Can you work these out from the model? Positions are in its coordinate system, mm. A direction names the side the tool comes from. Give positions to 0.01 mm unless a question says otherwise; leave off trailing zeros. Loops run counter-clockwise (first coordinate to the right, second up) from the corner with the lowest first, then second, coordinate; pieces in that order, holes last. Notation, with made-up numbers: (12, 8.5) - (35, 8.5) arc R20 cw to (35, 14.5) - close; hole circle Ø1 at (55.5, 32). An arc over 180 degrees is marked (long way). Answer in a Markdown table with one row per item.
from build123d import *

# Parameters (mm, degrees)
SKETCH1_W                                    = 130.62
SKETCH1_H                                    = 3
SKETCH1_W_2                                  = 18.99
SKETCH1_W_3                                  = 25.43
SKETCH1_W_4                                  = 84.2
SKETCH1_H_2                                  = 2.79860344
BOSS_EXTRUDE1_DEPTH                          = 2
SKETCH2_W                                    = 130.62
SKETCH2_H                                    = 178.45860344
BOSS_EXTRUDE2_DEPTH                          = 3
CSK_FOR_M3_COUNTERSUNK_FLAT_HEAD_SCR_2_COUNT = 2
CSK_FOR_M3_COUNTERSUNK_FLAT_HEAD_SCR_2_PITCH = 53.025276991
CSK_FOR_M3_COUNTERSUNK_FLAT_HEAD_SCR_3_COUNT = 2
CSK_FOR_M3_COUNTERSUNK_FLAT_HEAD_SCR_3_PITCH = 66.620192134
CSK_FOR_M3_COUNTERSUNK_FLAT_HEAD_SCR_4_COUNT = 2
CSK_FOR_M3_COUNTERSUNK_FLAT_HEAD_SCR_4_PITCH = 48.217527933
SKETCH9_W                                    = 2.047760895
SKETCH9_H                                    = 53.7
SKETCH9_W_2                                  = 2
BOSS_EXTRUDE3_DEPTH                          = 24
SKETCH10_W                                   = 130.62
SKETCH10_H                                   = 3
BOSS_EXTRUDE4_DEPTH                          = 22
CUT_EXTRUDE1_DEPTH                           = 22
BOSS_EXTRUDE5_DEPTH                          = 22
SKETCH13_R                                   = 2
BOSS_EXTRUDE6_DEPTH                          = 24.5
SKETCH15_W                                   = 126.572239105
SKETCH15_H                                   = 3
SKETCH15_W_2                                 = 2
SKETCH15_H_2                                 = 172.45860344
SKETCH15_W_3                                 = 2.047760895
BOSS_EXTRUDE7_DEPTH                          = 2.5


with BuildPart() as part:
    # Sketch1 → Boss-Extrude1 (new body)
    with BuildSketch(Plane(origin=(0, 0, 0), x_dir=(1, 0, 0), z_dir=(0, 1, 0))):
        with Locations((69.266788991, -134.782980897)):
            Rectangle(SKETCH1_W, SKETCH1_H)
        with Locations((69.266788991, -78.082980897)):
            Rectangle(SKETCH1_W, SKETCH1_H)
        Polygon((134.576788991, -20.082980897), (109.146788991, -20.082980897), (109.146788991, -67.500327372), (109.146788991, -76.582980897), (134.576788991, -76.582980897), align=None)
        Polygon((22.946788991, -33.891997438), (22.946788991, -20.082980897), (3.956788991, -20.082980897), (3.956788991, -76.582980897), (22.946788991, -76.582980897), align=None)
        Polygon((22.946788991, -17.082980897), (22.946788991, 39.175622543), (6.956788991, 39.175622543), (3.956788991, 39.175622543), (3.956788991, -17.082980897), align=None)
        Polygon((131.576788991, 39.175622543), (109.146788991, 39.175622543), (109.146788991, -17.082980897), (134.576788991, -17.082980897), (134.576788991, 39.175622543), align=None)
        with Locations((13.451788991, -18.582980897)):
            Rectangle(SKETCH1_W_2, SKETCH1_H)
        with Locations((121.861788991, -18.582980897)):
            Rectangle(SKETCH1_W_3, SKETCH1_H)
        with Locations((66.046788991, -18.683679177)):
            Rectangle(SKETCH1_W_4, SKETCH1_H_2)
        Polygon((23.946788991, 39.175622543), (108.146788991, 39.175622543), (109.146788991, 39.175622543), (131.576788991, 39.175622543), (134.576788991, 39.175622543), (134.576788991, 42.175622543), (3.956788991, 42.175622543), (3.956788991, 39.175622543), (6.956788991, 39.175622543), (22.946788991, 39.175622543), align=None)
    extrude(amount=BOSS_EXTRUDE1_DEPTH)

    # Sketch2 → Boss-Extrude2 (add)
    with BuildSketch(Plane.XZ):
        with Locations((69.266788991, 47.053679177)):
            Rectangle(SKETCH2_W, SKETCH2_H)
    extrude(amount=BOSS_EXTRUDE2_DEPTH)

    # Sketch8 → CSK for M3 Countersunk Flat Head Screw1 (revolve, cut)
    with BuildSketch(Plane(origin=(88.234088991, 0, 130.282980897), x_dir=(0, 0, 1), z_dir=(1, 0, 0))):
        Polygon((0, 0), (0, 3), (1.7, 3), (1.7, 1.45), (3.15, 0), align=None)
    csk_for_m3_countersunk_flat_head_screw1 = revolve(axis=Axis((88.234088991, 6.35, 130.282980897), (0, -1, 0)), mode=Mode.SUBTRACT)

    # CSK for M3 Countersunk Flat Head Scr 2: CSK for M3 Countersunk Flat Head Screw1 ×2
    with Locations(*[Vector(-0.958033656445997, 0, -0.2866557397239995) * (i * CSK_FOR_M3_COUNTERSUNK_FLAT_HEAD_SCR_2_PITCH) for i in range(1, CSK_FOR_M3_COUNTERSUNK_FLAT_HEAD_SCR_2_COUNT)]):
        add(csk_for_m3_countersunk_flat_head_screw1, mode=Mode.SUBTRACT)

    # CSK for M3 Countersunk Flat Head Scr 3: CSK for M3 Countersunk Flat Head Screw1 ×2
    with Locations(*[Vector(-0.762531574476027, 0, -0.6469510011794644) * (i * CSK_FOR_M3_COUNTERSUNK_FLAT_HEAD_SCR_3_PITCH) for i in range(1, CSK_FOR_M3_COUNTERSUNK_FLAT_HEAD_SCR_3_COUNT)]):
        add(csk_for_m3_countersunk_flat_head_screw1, mode=Mode.SUBTRACT)

    # CSK for M3 Countersunk Flat Head Scr 4: CSK for M3 Countersunk Flat Head Screw1 ×2
    with Locations(*[Vector(0.02696114993281913, 0, -0.9996364821245272) * (i * CSK_FOR_M3_COUNTERSUNK_FLAT_HEAD_SCR_4_PITCH) for i in range(1, CSK_FOR_M3_COUNTERSUNK_FLAT_HEAD_SCR_4_COUNT)]):
        add(csk_for_m3_countersunk_flat_head_screw1, mode=Mode.SUBTRACT)

    # Sketch9 → Boss-Extrude3 (add)
    with BuildSketch(Plane(origin=(0, 0, 0), x_dir=(1, 0, 0), z_dir=(0, 1, 0))):
        with Locations((133.552908543, -106.432980897)):
            Rectangle(SKETCH9_W, SKETCH9_H)
        with Locations((4.956788991, -106.432980897)):
            Rectangle(SKETCH9_W_2, SKETCH9_H)
    extrude(amount=BOSS_EXTRUDE3_DEPTH)

    # Sketch10 → Boss-Extrude4 (add)
    with BuildSketch(Plane(origin=(0, 2, 0), x_dir=(1, 0, 0), z_dir=(0, 1, 0))):
        with Locations((69.266788991, -134.782980897)):
            Rectangle(SKETCH10_W, SKETCH10_H)
    extrude(amount=BOSS_EXTRUDE4_DEPTH)

    # Sketch11 → Cut-Extrude1 (cut)
    with BuildSketch(Plane(origin=(134.576788991, 0, 0), x_dir=(0, 0, -1), z_dir=(1, 0, 0))):
        with BuildLine():
            Line((-126.332980897, 2), (-107.932980897, 2))
            Line((-107.932980897, 2), (-107.932980897, 12))
            Line((-107.932980897, 12), (-123.378368558, 12))
            ThreePointArc((-123.378368558, 12), (-125.578874654, 7.213677543), (-126.332980897, 2))
        make_face()
        with BuildLine():
            Line((-107.932980897, 2), (-89.532980897, 2))
            ThreePointArc((-89.532980897, 2), (-90.28708714, 7.213677543), (-92.487593236, 12))
            Line((-92.487593236, 12), (-107.932980897, 12))
            Line((-107.932980897, 12), (-107.932980897, 2))
        make_face()
    extrude(amount=-CUT_EXTRUDE1_DEPTH, mode=Mode.SUBTRACT)

    # Sketch12 → Boss-Extrude5 (add)
    with BuildSketch(Plane(origin=(0, 2, 0), x_dir=(1, 0, 0), z_dir=(0, 1, 0))):
        Polygon((134.576788991, 42.175622543), (3.956788991, 42.175622543), (3.956788991, -79.582980897), (5.956788991, -79.582980897), (5.956788991, 39.175622543), (132.529028096, 39.175622543), (132.529028096, -79.582980897), (134.576788991, -79.582980897), align=None)
    extrude(amount=BOSS_EXTRUDE5_DEPTH)

    # Sketch13 → Boss-Extrude6 (add)
    with BuildSketch(Plane(origin=(0, 0, 0), x_dir=(1, 0, 0), z_dir=(0, 1, 0))):
        with BuildLine():
            Line((125.229028096, -117.857980897), (125.229028096, -119.857980897))
            Line((125.229028096, -119.857980897), (125.229028096, -121.857980897))
            ThreePointArc((125.229028096, -121.857980897), (126.643241659, -121.272194459), (127.229028096, -119.857980897))
            ThreePointArc((127.229028096, -119.857980897), (126.643241659, -118.443767335), (125.229028096, -117.857980897))
        make_face()
        with BuildLine():
            ThreePointArc((125.229028096, -117.857980897), (123.814814534, -118.443767335), (123.229028096, -119.857980897))
            Line((123.229028096, -119.857980897), (125.229028096, -119.857980897))
            Line((125.229028096, -119.857980897), (125.229028096, -117.857980897))
        make_face()
        with BuildLine():
            Line((125.229028096, -119.857980897), (123.229028096, -119.857980897))
            ThreePointArc((123.229028096, -119.857980897), (123.814814534, -121.272194459), (125.229028096, -121.857980897))
            Line((125.229028096, -121.857980897), (125.229028096, -119.857980897))
        make_face()
        with BuildLine():
            ThreePointArc((125.229028096, -117.857980897), (123.814814534, -118.443767335), (123.229028096, -119.857980897))
            Line((123.229028096, -119.857980897), (125.229028096, -119.857980897))
            Line((125.229028096, -119.857980897), (125.229028096, -117.857980897))
        make_face()
        with BuildLine():
            ThreePointArc((13.209288991, -121.857980897), (14.623502553, -121.272194459), (15.209288991, -119.857980897))
            Line((15.209288991, -119.857980897), (13.209288991, -119.857980897))
            Line((13.209288991, -119.857980897), (13.209288991, -121.857980897))
        make_face()
        with BuildLine():
            Line((13.209288991, -119.857980897), (15.209288991, -119.857980897))
            ThreePointArc((15.209288991, -119.857980897), (14.623502553, -118.443767335), (13.209288991, -117.857980897))
            Line((13.209288991, -117.857980897), (13.209288991, -119.857980897))
        make_face()
        with BuildLine():
            Line((13.209288991, -119.857980897), (15.209288991, -119.857980897))
            ThreePointArc((15.209288991, -119.857980897), (14.623502553, -118.443767335), (13.209288991, -117.857980897))
            Line((13.209288991, -117.857980897), (13.209288991, -119.857980897))
        make_face()
        with BuildLine():
            Line((13.209288991, -119.857980897), (13.209288991, -117.857980897))
            ThreePointArc((13.209288991, -117.857980897), (11.209288991, -119.857980897), (13.209288991, -121.857980897))
            Line((13.209288991, -121.857980897), (13.209288991, -119.857980897))
        make_face()
        with BuildLine():
            ThreePointArc((15.209288991, -93.007980897), (14.623502553, -91.593767335), (13.209288991, -91.007980897))
            Line((13.209288991, -91.007980897), (13.209288991, -93.007980897))
            Line((13.209288991, -93.007980897), (15.209288991, -93.007980897))
        make_face()
        with BuildLine():
            ThreePointArc((13.209288991, -95.007980897), (14.623502553, -94.422194459), (15.209288991, -93.007980897))
            Line((15.209288991, -93.007980897), (13.209288991, -93.007980897))
            Line((13.209288991, -93.007980897), (13.209288991, -95.007980897))
        make_face()
        with BuildLine():
            ThreePointArc((15.209288991, -93.007980897), (14.623502553, -91.593767335), (13.209288991, -91.007980897))
            Line((13.209288991, -91.007980897), (13.209288991, -93.007980897))
            Line((13.209288991, -93.007980897), (15.209288991, -93.007980897))
        make_face()
        with BuildLine():
            ThreePointArc((13.209288991, -95.007980897), (14.623502553, -94.422194459), (15.209288991, -93.007980897))
            Line((15.209288991, -93.007980897), (13.209288991, -93.007980897))
            Line((13.209288991, -93.007980897), (13.209288991, -95.007980897))
        make_face()
        with BuildLine():
            Line((13.209288991, -93.007980897), (13.209288991, -91.007980897))
            ThreePointArc((13.209288991, -91.007980897), (11.209288991, -93.007980897), (13.209288991, -95.007980897))
            Line((13.209288991, -95.007980897), (13.209288991, -93.007980897))
        make_face()
        with Locations(Location((125.229028096, -93.007980897, 0), (0, 0, 90))):
            Circle(SKETCH13_R)
    extrude(amount=BOSS_EXTRUDE6_DEPTH)

    # Sketch15 → Boss-Extrude7 (add)
    with BuildSketch(Plane(origin=(0, 24, 0), x_dir=(1, 0, 0), z_dir=(0, 1, 0))):
        with Locations((69.242908544, 40.675622543)):
            Rectangle(SKETCH15_W, SKETCH15_H)
        with Locations((4.956788991, -47.053679177)):
            Rectangle(SKETCH15_W_2, SKETCH15_H_2)
        with Locations((4.956788991, 40.675622543)):
            Rectangle(SKETCH15_W_2, SKETCH15_H)
        with Locations((133.552908543, 40.675622543)):
            Rectangle(SKETCH15_W_3, SKETCH15_H)
        Polygon((134.576788991, -136.282980897), (134.576788991, 39.175622543), (132.529028096, 39.175622543), (132.529028096, -133.282980897), (132.529028096, -136.282980897), align=None)
        with Locations((4.956788991, -134.782980897)):
            Rectangle(SKETCH15_W_2, SKETCH15_H)
        with Locations((69.242908544, -134.782980897)):
            Rectangle(SKETCH15_W, SKETCH15_H)
    extrude(amount=BOSS_EXTRUDE7_DEPTH)


solid = part.part
Q1. Imagine slicing it at B-B, the plane y = 16.5. Write out the boundary of the cut face in (x, z), and give its area (3 significant figures).
Checked values:
| item | result |
|---|---|
| outline | (3.96, -42.18) - (134.58, -42.18) - (134.58, 136.28) - (3.96, 136.28) - close; circle Ø4 at (13.21, 93.01); circle Ø4 at (13.21, 119.86); circle Ø4 at (125.23, 93.01); circle Ø4 at (125.23, 119.86); hole (5.96, -39.18) - (132.53, -39.18) - (132.53, 133.28) - (5.96, 133.28) - close |
| area | 1,530 mm² |
Q2. If we mould it in two halves opening along X, with no side actions, what happens to faces 3 (the face through (68, 13, -39.176)), 4 (the face through (134.577, 12, 48)), 5 (the face through (68, -3, 48)), 6 (the face through (37.359, -2.214, 85.485))? For each: released by +X, released by -X, zero draft, split by the parting line, or undercut.
Checked values:
| item | result |
|---|---|
| face 3 | undercut |
| face 4 | released by +X |
| face 5 | zero draft |
| face 6 | undercut |
Q3. Imagine slicing it at C-C, the plane y = 8. Write out the boundary of the cut face in (x, z), and give its area (3 significant figures).
Checked values:
| item | result |
|---|---|
| outline | (3.96, -42.18) - (134.58, -42.18) - (134.58, 90.54) - (132.53, 90.54) - (132.53, -39.18) - (5.96, -39.18) - (5.96, 133.28) - (132.53, 133.28) - (132.53, 125.33) - (134.58, 125.33) - (134.58, 136.28) - (3.96, 136.28) - close; circle Ø4 at (13.21, 93.01); circle Ø4 at (13.21, 119.86); circle Ø4 at (125.23, 93.01); circle Ø4 at (125.23, 119.86) |
| area | 1,460 mm² |
Q4. For pin 1 (8 mm diameter, centred on x = 116.5, z = 109, fed in from +Y); pin 2 (2 mm diameter, centred on x = 86, z = 77, fed in from +Y); pin 3 (2 mm diameter, centred on x = 126, z = 93.5, fed in from +Y), each with a flat end and sliding along its axis, tell me the tip position at first contact or that it passes through.
Checked values:
| item | result |
|---|---|
| pin 1 | stops at y = 0 |
| pin 2 | stops at y = 2 |
| pin 3 | stops at y = 24.5 |
Q5. Imagine slicing it at A-A, the plane z = 106.5. Write out the boundary of the cut face in (x, y), and give its area (3 significant figures).
Checked values:
| item | result |
|---|---|
| outline | (3.96, -3) - (134.58, -3) - (134.58, 2) - (132.53, 2) - (132.53, 0) - (5.96, 0) - (5.96, 26.5) - (3.96, 26.5) - close; (132.53, 12) - (134.58, 12) - (134.58, 26.5) - (132.53, 26.5) - close |
| area | 479 mm² |
Q6. On a 3-axis mill with a long thin cutter (end or side, diameter ignored), from which of +Z, -Z, +X, -X, +Y, -Y can I reach the whole of each face in a straight line? I mean faces 1 (the face through (13, 24.5, 120)), 2 (the face through (88.89, -2.21, 131.85)). Say none if no direction works.
Checked values:
| item | result |
|---|---|
| face 1 | +Y |
| face 2 | +Y, -Y |
Q7. If I drill on line 1 (Z direction, x = 123, y = 7.5); line 2 (X direction, y = 8.25, z = 1.5); line 3 (X direction, y = 9, z = 91.5), over which ranges is the centre line in solid material (lowest first)? Write a range as [from, to].
Checked values:
| item | result |
|---|---|
| line 1 | z = [-42.18, -39.18], [133.28, 136.28] |
| line 2 | x = [3.96, 5.96], [132.53, 134.58] |
| line 3 | x = [3.96, 5.96], [11.9, 14.52], [123.92, 126.54] |
Q8. Imagine slicing it at D-D, the plane x = 103. Write out the boundary of the cut face in (y, z).
Checked values:
| item | result |
|---|---|
| outline | (-3, -42.18) - (26.5, -42.18) - (26.5, -39.18) - (0, -39.18) - (0, 17.28) - (2, 17.28) - (2, 20.08) - (0, 20.08) - (0, 76.58) - (2, 76.58) - (2, 79.58) - (0, 79.58) - (0, 133.28) - (26.5, 133.28) - (26.5, 136.28) - (-3, 136.28) - close |
